Model file for the job. Use its own axes, mm. Face numbers are marked on the shaded views. A direction names the side the tool comes from. Coordinates: 2 decimals unless noted, no trailing zeros. Write each loop counter-clockwise with the first axis right and the second up, starting at its lowest first coordinate (ties: lowest second). Pieces come first, ordered by that corner, then holes. Notation, with made-up numbers: (78, -28) - (86, -28) arc R22 cw to (86, -11) - close; hole circle Ø11 at (89.5, -4). An arc over 180 degrees is marked (long way). Put each result on its own line as item: value. Start each with the question number.
1. Drop flat-ended pins along their axis: P1, Ø6, axis at x = 0.5, z = -50, coming from the -Y side; P2, Ø8, axis at x = -1, y = -21, coming from the +Z side; P3, Ø10, axis at y = 1, z = -68, coming from the -X side. Give the stop position or say it passes through.
2. Saw through at B-B, the plane z = -42. Write the cut outline in (x, y), plus the area to 3 significant figures.
3. Saw through at D-D, the plane y = 23. Write the cut outline in (x, z).
4. Drill centre lines: L1, parallel to Y at x = 0, z = -125.5; L2, parallel to Z at x = -19, y = 22; L3, parallel to Y at x = -3, z = -82.5. Where is each one in solid material? Low to high. Write a range as from..to.
5. Which spindle directions (+Z, -Z, +X, -X, +Y, -Y) get a long thin tool onto all of the face, cutting with end or side? Do the marked faces 1 and 2. Say none if no direction does.
6. Saw through at A-A, the plane x = 17.5. Write the cut outline in (y, z).
7. Saw through at C-C, the plane y = -25. Write the cut outline in (x, z).
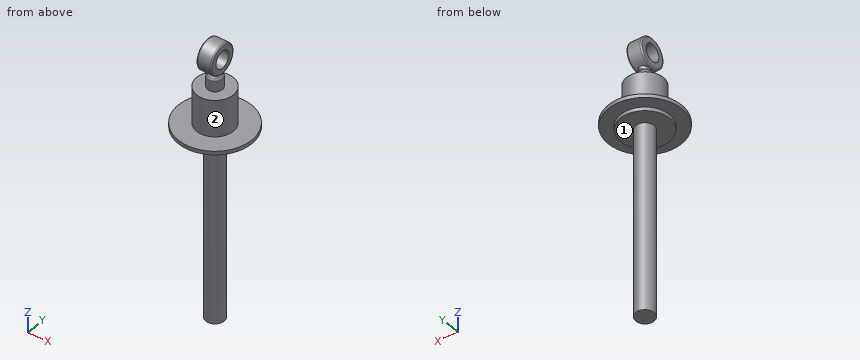
```python
from build123d import *

# Parameters (mm, degrees)
SKETCH1_W           = 7.5
SKETCH1_H           = 154
SKETCH2_4_R         = 12
SKETCH2_4_R_2       = 7
BOSS_EXTRUDE1_DEPTH = 6
FILLET1_R           = 1
FILLET2_R           = 2


with BuildPart() as part:
    # Sketch1 → Revolve1 (revolve)
    with BuildSketch(Plane.YZ, mode=Mode.PRIVATE) as revolve1_sk:
        with Locations((3.75, -80)):
            Rectangle(SKETCH1_W, SKETCH1_H)
        Polygon((6, 43), (0, 43), (0, 0), (20, 0), (30, 0), (30, 3), (15, 3), (15, 33), (6, 33), align=None)
        Polygon((20, 0), (0, 0), (0, -3), (7.5, -3), (20, -3), align=None)
    revolve(revolve1_sk.sketch.rotate(Axis((0, 0, 49.693213244), (0, 0, -1)), 90), axis=Axis((0, 0, 49.693213244), (0, 0, -1)))

    # Sketch2 → Revolve2 (revolve)
    with BuildSketch(Plane.YZ, mode=Mode.PRIVATE) as revolve2_sk:
        with BuildLine():
            ThreePointArc((5.142857143, 46.807015806), (2.63579798, 45.942165309), (0, 45.649110641))
            Line((0, 45.649110641), (0, 43))
            Line((0, 43), (6, 43))
            ThreePointArc((6, 43), (4.048842445, 44.560700337), (5.142857143, 46.807015806))
        make_face()
    revolve(revolve2_sk.sketch.rotate(Axis((0, 0, 57.649110641), (0, 0, -1)), 90), axis=Axis((0, 0, 57.649110641), (0, 0, -1)))

    # Sketch2_4 → Boss-Extrude1 (add, symmetric)
    with BuildSketch(Plane.YZ):
        with Locations(Location((0, 57.649110641, 0), (0, 0, 270))):
            Circle(SKETCH2_4_R)
        with Locations(Location((0, 57.649110641, 0), (0, 0, 270))):
            Circle(SKETCH2_4_R_2, mode=Mode.SUBTRACT)
    extrude(amount=BOSS_EXTRUDE1_DEPTH, both=True)

    # Fillet1
    fillet1_edges = [part.edges().sort_by_distance(p)[0] for p in [
        (-6, 0, 69.649110641),
        (6, 0, 69.649110641),
    ]]
    fillet(fillet1_edges, radius=FILLET1_R)

    # Fillet2
    fillet2_edges = [part.edges().sort_by_distance(p)[0] for p in [
        (-6, 0, 43),
    ]]
    fillet(fillet2_edges, radius=FILLET2_R)


solid = part.part
```
Final values:
1. P1: stops at y = -7.5
1. P2: stops at z = 3
1. P3: stops at x = -7.5
2. outline: circle Ø15 at (0, 0)
2. area: 177 mm²
3. outline: (-19.26, 0) - (19.26, 0) - (19.26, 3) - (-19.26, 3) - close
4. L1: y = -7.5..7.5
4. L2: z = 0..3
4. L3: y = -6.87..6.87
5. face 1: -Z
5. face 2: +Z
6. outline: (-24.37, 0) - (-9.68, 0) - (-9.68, -3) - (9.68, -3) - (9.68, 0) - (24.37, 0) - (24.37, 3) - (-24.37, 3) - close
7. outline: (-16.58, 0) - (16.58, 0) - (16.58, 3) - (-16.58, 3) - close
